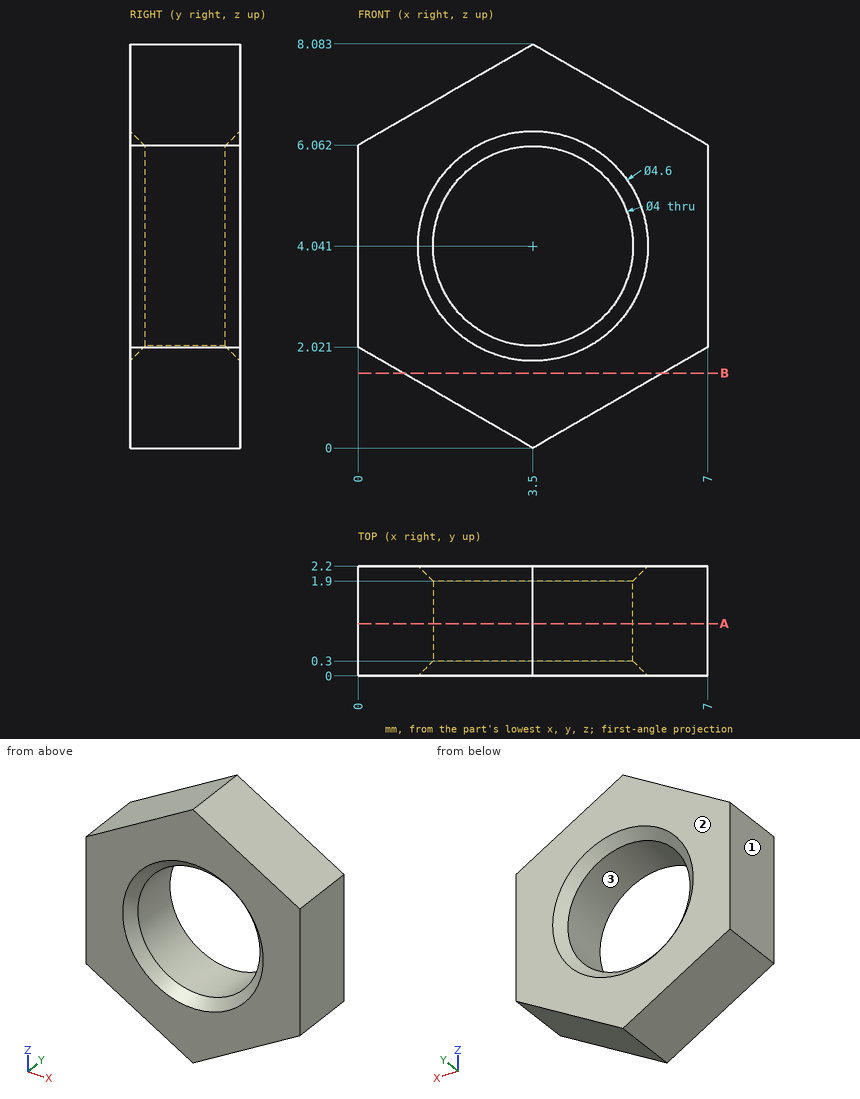
Here's the drawing with two shaded views (mm, measured from the low corner). I have some questions. Give positions to 0.01 mm unless a question says otherwise; leave off trailing zeros. Loops run counter-clockwise (first coordinate to the right, second up) from the corner with the lowest first, then second, coordinate; pieces in that order, holes last. Notation, with made-up numbers: (9, 35.5) - (26, 35.5) arc R7 ccw to (26, 47.5) - close; hole circle Ø10 at (7.25, 13.25). An arc over 180 degrees is marked (long way). One line per item, written item: value.
(1) If we section it at A-A, the plane y = 1.05: List the corners of the cut face in (x, z) for me.
Verdict:
outline: (0, 2.02) - (3.5, 0) - (7, 2.02) - (7, 6.06) - (3.5, 8.08) - (0, 6.06) - close; hole circle Ø4 at (3.5, 4.04)
(2) If we mould it in two halves opening along X, with no side actions, what happens to the marked faces 1, 2 and 3? For each: released by +X, released by -X, zero draft, split by the parting line, or undercut.
Verdict:
face 1: released by -X
face 2: zero draft
face 3: undercut
(3) I need wall thicknesses on line 1 along X through (y, z) = (0.9, 4); line 2 along X through (y, z) = (1.65, 5) (1 decimal); line 3 along Z through (x, y) = (2.5, 0.4) (1 decimal). Which ranges of each line are inside material? Lowest first, please.
Verdict:
line 1: 0 to 1.5, 5.5 to 7
line 2: 0 to 1.7, 5.3 to 7
line 3: 0.6 to 2.3, 5.8 to 7.5
(4) If we section it at B-B, the plane z = 1.5: List the corners of the cut face in (x, y) for me.
Verdict:
outline: (0.9, 0) - (6.1, 0) - (6.1, 2.2) - (0.9, 2.2) - close
(5) I'm going to push a flat-ended pin straight in: pin 1 (3 mm diameter, centred on x = 4.5, z = 2.5, fed in from -Y). Where does the tip first touch, or does it pass through?
Verdict:
pin 1: y = 0
